Part print with two shaded views. Sizes in mm from the minimum x, y, z corner. Give positions to 0.01 mm unless a question says otherwise; leave off trailing zeros. Write each loop counter-clockwise with the first axis right and the second up, starting at its lowest first coordinate (ties: lowest second). Pieces come first, ordered by that corner, then holes. Notation, with made-up numbers: M 71.25,-35.75 L 86.25,-35.75 A6 cw 86.25,-30.75 Z; hole C 38,34 d4. An arc over 180 degrees is marked long. Return JSON: item names as keys, results as strings. Group by question number.
Q1. Band-saw the part on C-C, the plane z = 2.3. Count the separate pieces of the cut face and the enclosed holes in it, then the cut area to 3 significant figures.
Q2. Flat gauge pins, fed straight in: pin 1 Ø1.5 at (y, z) = (7, 4) entering from -X; pin 2 Ø1 at (y, z) = (2.5, 1) entering from -X; pin 3 Ø4 at (x, y) = (4.73, 4.31) entering from +Z. Where does each tip first touch, or does it go through?
Q3. Band-saw the part on A-A, the plane x = 4.5. Give the cut face in (y, z).
Q4. Band-saw the part on D-D, the plane x = 24.5. Give the cut face in (y, z).
Q5. Pull direction Y, two halves, no side cores. Call the marked faces 1, 2 and 3: +Y half, -Y half, draft (parallel to the pull), parting line (faces both ways), or undercut.
Q6. Band-saw the part on B-B, the plane y = 2.25. Give the cut face in (x, z), then the cut area to 3 significant figures.
Q7. Wall check: probe 1 along X at (y, z) = (6.5, 4.75) (1 decimal); probe 2 along X at (y, z) = (6, 2.3) (1 decimal); probe 3 along Y at (x, z) = (26.5, 0.45). Give the ranges that are in metal, low to high.
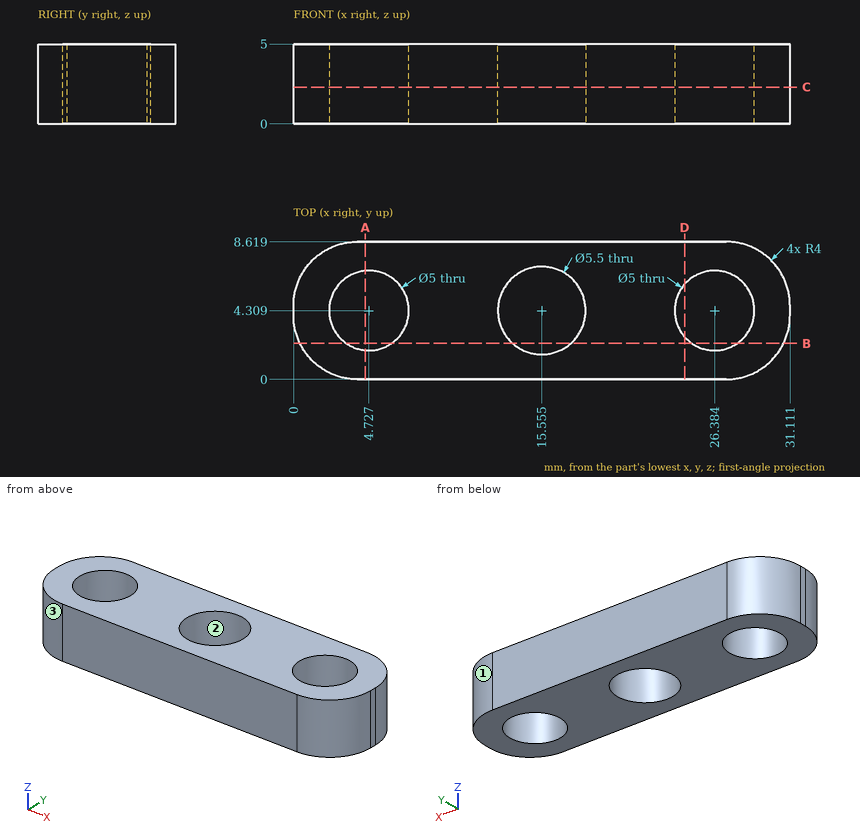
From the geometry:
{
 "1": {"separate pieces": "1", "enclosed holes": "3", "area": "191 mm^2"},
 "2": {"pin 1": "stops at x = 0.35", "pin 2": "stops at x = 0.13", "pin 3": "passes through"},
 "3": {"outline": "M 0,0 L 1.82,0 L 1.82,5 L 0,5 Z; M 6.8,0 L 8.62,0 L 8.62,5 L 6.8,5 Z"},
 "4": {"outline": "M 0,0 L 2.67,0 L 2.67,5 L 0,5 Z; M 5.95,0 L 8.62,0 L 8.62,5 L 5.95,5 Z"},
 "5": {"face 1": "+Y half", "face 2": "undercut", "face 3": "-Y half"},
 "6": {"outline": "M 0.4,0 L 3.31,0 L 3.31,5 L 0.4,5 Z; M 6.14,0 L 13.73,0 L 13.73,5 L 6.14,5 Z; M 17.38,0 L 24.97,0 L 24.97,5 L 17.38,5 Z; M 27.8,0 L 30.71,0 L 30.71,5 L 27.8,5 Z", "area": "105 mm^2"},
 "7": {"probe 1": "x = 0.5 to 3.5, 5.9 to 13.9, 17.2 to 25.2, 27.6 to 30.6", "probe 2": "x = 0.2 to 2.9, 6.6 to 13.4, 17.7 to 24.5, 28.2 to 30.9", "probe 3": "y = 0 to 1.81, 6.81 to 8.62"}
}
